Source: CAD feature listing. Evaluate the final solid. Frame: model axes, mm. Face numbers are marked on the shaded views. Round coordinates to 2 decimals unless told otherwise and drop trailing zeros. Loops run counter-clockwise (first coordinate to the right, second up) from the corner with the lowest first, then second, coordinate; pieces in that order, holes last.
(1) Section D-D, the plane y = -0.75. Return the cut outline in (x, z), plus the area to 3 significant figures.
(2) Section B-B, the plane y = 3.25. Return the cut outline in (x, z), plus the area to 3 significant figures.
(3) First-contact query: pin 1 Ø6 at (x, y) = (16.5, 4.5) entering from -Z; pin 2 Ø6 at (x, y) = (-6, 4) entering from +Z; pin 3 Ø5 at (y, z) = (5, -21) entering from +X. Flat tips, straight axial feed; report the tip coordinate or a pass-through.
(4) Mould query, pull axis Z, two halves, no side actions, for the marked faces 1, 2 and 3. Classes: pulls with the +Z half, pulls with the -Z half, needs draft (parallel to the pull), parting line crosses it, or undercut.
(5) Section A-A, the plane x = 0. Return the cut outline in (y, z).
(6) Section C-C, the plane z = 0. Count the separate pieces of the cut face and the enclosed holes in it, plus the area to 3 significant figures.
(7) Material intervals for probe 1 along Z at (x, y) = (0, 5.75); probe 2 along Y at (x, z) = (14, -22); probe 3 along Z at (x, y) = (-8, 5), sorted ascending.
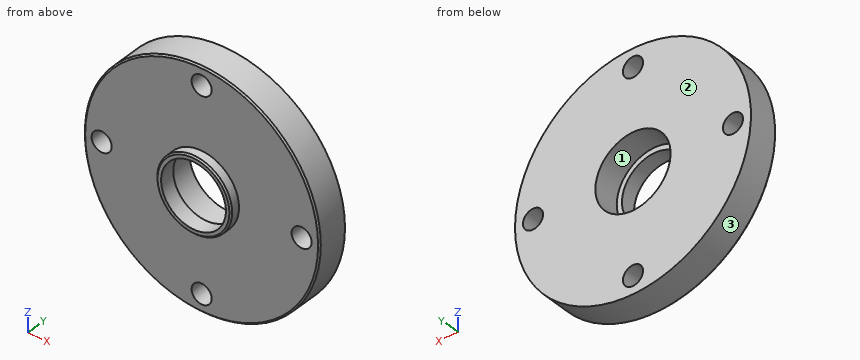
```python
from build123d import *

# Parameters (mm, degrees)
SKETCH2_R                                = 9.50595
BOSS_EXTRUDE1_DEPTH                      = 2.159
SKETCH3_R                                = 9.50595
BOSS_EXTRUDE2_DEPTH                      = 0.381
BOSS_EXTRUDE2_TAPER                      = 45
HOLE1_D                                  = 5.1054
HOLE1_DEPTH                              = 7.9375
HOLE2_D                                  = 5.1054
HOLE2_DEPTH                              = 10.4775
CBORE_FOR_M14_HEX_HEAD_BOLT1_D           = 16.4719
CBORE_FOR_M14_HEX_HEAD_BOLT1_DEPTH       = 10.4775
CBORE_FOR_M14_HEX_HEAD_BOLT1_CBORE_D     = 19.1008
CBORE_FOR_M14_HEX_HEAD_BOLT1_CBORE_DEPTH = 6.6675


with BuildPart() as part:
    # Sketch1 → Revolve1 (revolve)
    with BuildSketch(Plane(origin=(0, 0, 0), x_dir=(-1, 0, 0), z_dir=(0, 0, -1))):
        Polygon((-29.591, 0), (0, 0), (0, 7.9375), (-29.972, 7.9375), (-29.972, 0.381), align=None)
    revolve(axis=Axis((0, 0, 0), (0, 1, 0)))

    # Sketch2 → Boss-Extrude1 (add)
    with BuildSketch(Plane.XZ):
        Circle(SKETCH2_R)
    extrude(amount=BOSS_EXTRUDE1_DEPTH)

    # Sketch3 → Boss-Extrude2 (add)
    with BuildSketch(Plane.XZ.offset(2.159)):
        Circle(SKETCH3_R)
    extrude(amount=BOSS_EXTRUDE2_DEPTH, taper=BOSS_EXTRUDE2_TAPER)

    # Hole1
    with Locations(Plane(origin=(0, 0, 0), x_dir=(-1, 0, 0), z_dir=(0, -1, 0))):
        with Locations((0, -25.4)):
            Hole(HOLE1_D / 2, depth=HOLE1_DEPTH)

    # Hole2
    with Locations(Plane(origin=(0, 7.9375, 0), x_dir=(1, 0, 0), z_dir=(0, 1, 0))):
        with Locations((0, 25.4), (25.4, 0), (-25.4, 0)):
            Hole(HOLE2_D / 2, depth=HOLE2_DEPTH)

    # CBORE for M14 Hex Head Bolt1
    with Locations(Plane(origin=(0, 7.9375, 0), x_dir=(1, 0, 0), z_dir=(0, 1, 0))):
        with Locations((0, 0)):
            CounterBoreHole(CBORE_FOR_M14_HEX_HEAD_BOLT1_D / 2, CBORE_FOR_M14_HEX_HEAD_BOLT1_CBORE_D / 2, CBORE_FOR_M14_HEX_HEAD_BOLT1_CBORE_DEPTH, depth=CBORE_FOR_M14_HEX_HEAD_BOLT1_DEPTH)


solid = part.part
```
Output values:
1. outline: circle Ø19.01 at (0, 0); hole circle Ø16.47 at (0, 0)
1. area: 70.8 mm2
2. outline: circle Ø59.94 at (0, 0); hole circle Ø5.11 at (-25.4, 0); hole circle Ø19.1 at (0, 0); hole circle Ø5.11 at (0, -25.4); hole circle Ø5.11 at (0, 25.4); hole circle Ø5.11 at (25.4, 0)
2. area: 2,450 mm2
3. pin 1: stops at z = -26.76
3. pin 2: stops at z = 29.82
3. pin 3: stops at x = 23.58
4. face 1: undercut
4. face 2: needs draft
4. face 3: parting line crosses it
5. outline: (-2.54, -9.12) - (-2.16, -9.51) - (0, -9.51) - (0, -22.85) - (7.94, -22.85) - (7.94, -9.55) - (1.27, -9.55) - (1.27, -8.24) - (-2.54, -8.24) - close; (-2.54, 8.24) - (1.27, 8.24) - (1.27, 9.55) - (7.94, 9.55) - (7.94, 22.85) - (0, 22.85) - (0, 9.51) - (-2.16, 9.51) - (-2.54, 9.12) - close; (0, -29.59) - (0.38, -29.97) - (7.94, -29.97) - (7.94, -27.95) - (0, -27.95) - close; (0, 27.95) - (7.94, 27.95) - (7.94, 29.97) - (0.38, 29.97) - (0, 29.59) - close
6. separate pieces: 4
6. enclosed holes: 0
6. area: 253 mm2
7. probe 1: z = -29.97 to -27.95, -22.85 to -9.55, 9.55 to 22.85, 27.95 to 29.97
7. probe 2: y = 0 to 7.94
7. probe 3: z = -28.88 to -5.22, 5.22 to 28.88
